Can you work these out from the model? Positions are in its coordinate system, mm. A direction names the side the tool comes from. Round coordinates to 2 decimals unless told otherwise and drop trailing zeros. Order: outer loops, then holes, each group sorted by start corner. A loop starts at its lowest first (then second) coordinate and runs counter-clockwise, first axis right, second up.
Q1. If we section it at B-B (z = 8.5): Please give me the cut outline in (x, y).
Q2. If we section it at C-C (z = -7): Please give me the cut outline in (x, y), plus the area to 3 significant figures.
Q3. If we section it at D-D (x = -14): Please give me the cut outline in (y, z), plus the area to 4 significant figures.
Q4. If I drill on line 1 (X direction, y = 2, z = 1.25); line 2 (X direction, y = 13.5, z = 13.75); line 3 (X direction, y = 18.5, z = -7.5), over which ranges is the centre line in solid material (lowest first)?
Q5. For faces 5 (the face through (-34, 14, -10.57)), 6 (the face through (32, 14, -10.57)), 7 (the face through (-25, 8, 13.82)), 8 (the face through (-2, 8, 15.57)), 9 (the face through (-18, 10, 11)), which set-ups out of +Z, -Z, +X, -X, +Y, -Y let a thin tool reach every point of the face, with its end or its side?
Q6. We'd pull the mould along X, two halves only. Please class faces 1 (the face through (30.72, 6.88, -12.05)), 2 (the face through (-2, -3, 1)), 3 (the face through (25, 10, -3.18)), 4 (the face through (-25, 8, -1.68)): pulls with the +X half, pulls with the -X half, needs draft (parallel to the pull), parting line crosses it, or undercut.
Q7. If we section it at A-A (x = 25.5): Please give me the cut outline in (y, z), plus the area to 3 significant figures.
Q8. Will these pins go through, and if not, where does the flat tip stop? P1, Ø1.3, axis at x = -23.5, y = 13.5, coming from the -Z side; P2, Ø3, axis at x = -4, z = 4.5, coming from the +Y side; P3, Ø1.3, axis at x = 20.5, y = 12.5, coming from the -Z side; P4, Ø3.5, axis at x = -35.5, y = 7, coming from the +Z side.
Autodesk Inventor part; units mm, degrees
ref_plane "YZ Plane" through (0, 0, 0) normal (1, 0, 0) x (0, 1, 0)
ref_plane "XZ Plane" through (0, 0, 0) normal (0, 1, 0) x (-1, 0, 0)
ref_plane "XY Plane" through (0, 0, 0) normal (0, 0, 1) x (1, 0, 0)
sketch "Boceto1" plane through (0, 0, 0) normal (0, 1, 0) x (-1, 0, 0)
  line L0 (24, 13.57) -> (26.5, 13.57)
  line L1 (-26.5, 13.57) -> (26.5, -13.57) construction
  line L2 (26.5, 13.57) -> (-26.5, -13.57) construction
  line L3 (24, 13.57) -> (24, 10.27) construction
  line L4 (24, 10.27) -> (20, 10.27) construction
  line L5 (20, 10.27) -> (20, 1.87) construction
  line L6 (20, 1.87) -> (24, 1.87) construction
  line L7 (24, 1.87) -> (24, -1.43) construction
  line L8 (24, -1.43) -> (26.5, -1.43) construction
  line L9 (26.75, -1.68) -> (23.75, -1.68)
  line L10 (23.75, -1.68) -> (23.75, 1.62)
  line L11 (23.75, 1.62) -> (19.5, 1.62)
  line L12 (19.5, 10.52) -> (23.75, 10.52)
  line L13 (23.75, 10.52) -> (23.75, 13.82)
  line L14 (27, 15.57) -> (0, 15.57)
  line L15 (18, 0.12) -> (22.25, 0.12)
  line L16 (22.25, 0.12) -> (22.25, -3.18)
  line L17 (22.25, -3.18) -> (26.75, -3.18)
  line L18 (18, 12.27) -> (0, 12.27)
  line L19 (19.5, 10.52) -> (18, 10.52)
  line L20 (19.5, 1.62) -> (18, 1.62)
  line L21 (27, 15.57) -> (29.75, 15.57)
  line L22 (29.75, 15.57) -> (29.75, -10.57)
  line L23 (29.75, -10.57) -> (36.3, -10.57)
  line L24 (36.3, -10.57) -> (36.3, -13.57)
  line L25 (36.3, -13.57) -> (26.75, -13.57)
  line L26 (0, 12.27) -> (0, 15.57)
  line L27 (23.75, 13.82) -> (26.75, 13.82)
  line L28 (18, 12.27) -> (18, 10.52)
  line L29 (18, 1.62) -> (18, 0.12)
  line L30 (26.75, -13.57) -> (26.75, -3.18)
  line L31 (26.75, -1.68) -> (26.75, 13.82)
  line L32 (26.5, 13.57) -> (26.5, -1.68) construction
  point P0 (0, 0)
  point P1 (23.75, 13.57)
  point P2 (0, 13.57)
  point P3 (27, -12.07)
  dimension "d1" = 27.14
  dimension "d2" = 15
  dimension "d4" = 3.3
  dimension "d5" = 4
  dimension "d6" = 3.3
  dimension "d10" = 0.25
  dimension "d11" = 0.25
  dimension "d12" = 1.5
  dimension "d16" = 3
  dimension "d17" = 29.14
  dimension "d23" = 18
  dimension "d24" = 2
  dimension "d25" = 0.25
  dimension "d27" = 15.57
  dimension "d28" = 29.75
  dimension "d29" = 3.3
  dimension "d30" = 0.25
  dimension "d31" = 20
  dimension "d32" = 6.5
  dimension "d33" = 0.25
  dimension "d34" = 4.25
  dimension "d36" = 0.25
  dimension "d51" = 36.3
extrude "Extrusión1" add sketch "Boceto1" along normal blind 20
mirror "Simetría1" about plane through (0, 0, 0) normal (1, 0, 0) of "Extrusión1"
sketch "Boceto2" plane through (0, 0, 0) normal (0, -1, 0) x (1, 0, 0)
  line L0 (18, 1.62) -> (18, 0.12)
  line L1 (18, 1.62) -> (-18, 1.62)
  line L2 (-18, 1.62) -> (-18, 0.12)
  line L3 (-18, 0.12) -> (-22.25, 0.12)
  line L4 (-22.25, 0.12) -> (-22.25, -3.18)
  line L5 (-22.25, -3.18) -> (-26.75, -3.18)
  line L6 (-26.75, -3.18) -> (-26.75, -13.57)
  line L7 (26.75, -3.18) -> (26.75, -13.57)
  line L8 (22.25, -3.18) -> (26.75, -3.18)
  line L9 (22.25, 0.12) -> (22.25, -3.18)
  line L10 (18, 0.12) -> (22.25, 0.12)
  line L11 (26.75, -13.57) -> (36.3, -13.57)
  line L12 (36.3, -13.57) -> (36.3, -10.57)
  line L13 (-36.3, -10.57) -> (-29.75, -10.57)
  line L14 (-36.3, -13.57) -> (-36.3, -10.57)
  line L15 (-26.75, -13.57) -> (-36.3, -13.57)
  line L16 (23.75, 1.62) -> (18, 1.62)
  line L17 (23.75, -1.68) -> (23.75, 1.62)
  line L18 (26.75, -1.68) -> (23.75, -1.68)
  line L19 (36.3, -10.57) -> (29.75, -10.57)
  line L20 (26.75, -1.68) -> (29.75, -1.68)
  line L21 (29.75, -10.57) -> (29.75, 15.57)
  line L22 (-23.75, 1.62) -> (-18, 1.62)
  line L23 (-23.75, -1.68) -> (-23.75, 1.62)
  line L24 (-26.75, -1.68) -> (-23.75, -1.68)
  line L25 (-26.75, 13.82) -> (-26.75, -1.68)
  line L26 (-26.75, -1.68) -> (-29.75, -1.68)
  line L27 (-29.75, -10.57) -> (-29.75, 15.57)
  line L28 (26.75, -13.57) -> (-26.75, -13.57)
  line L29 (-18, 12.27) -> (18, 12.27)
  line L30 (12.75, 12.27) -> (12.75, 1.62)
  line L31 (26.75, 13.82) -> (26.75, -1.68)
  line L32 (-29.75, 15.57) -> (29.75, 15.57)
  line L33 (-16.75, 12.27) -> (-16.75, 1.62)
  line L34 (23.75, 13.82) -> (26.75, 13.82)
  line L35 (18, 10.52) -> (23.75, 10.52)
  line L36 (23.75, 10.52) -> (23.75, 13.82)
  line L37 (18, 12.27) -> (18, 10.52)
  line L38 (-23.75, 10.52) -> (-23.75, 13.82)
  line L39 (-18, 10.52) -> (-23.75, 10.52)
  line L40 (-18, 12.27) -> (-18, 10.52)
  line L41 (-18, 12.27) -> (18, 12.27)
  line L42 (18, 12.27) -> (18, 10.52)
  line L43 (18, 10.52) -> (23.75, 10.52)
  line L44 (23.75, 10.52) -> (23.75, 13.82)
  line L45 (23.75, 13.82) -> (26.75, 13.82)
  line L46 (26.75, 13.82) -> (26.75, -1.68)
  line L47 (26.75, -1.68) -> (23.75, -1.68)
  line L48 (23.75, -1.68) -> (23.75, 1.62)
  line L49 (23.75, 1.62) -> (18, 1.62)
  line L50 (18, 1.62) -> (18, 0.12)
  line L51 (18, 0.12) -> (22.25, 0.12)
  line L52 (22.25, 0.12) -> (22.25, -3.18)
  line L53 (22.25, -3.18) -> (26.75, -3.18)
  line L54 (26.75, -3.18) -> (26.75, -13.57)
  line L55 (26.75, -13.57) -> (36.3, -13.57)
  line L56 (36.3, -13.57) -> (36.3, -10.57)
  line L57 (36.3, -10.57) -> (29.75, -10.57)
  line L58 (29.75, -10.57) -> (29.75, 15.57)
  line L59 (-29.75, 15.57) -> (29.75, 15.57)
  line L60 (-29.75, -10.57) -> (-29.75, 15.57)
  line L61 (-36.3, -10.57) -> (-29.75, -10.57)
  line L62 (-36.3, -13.57) -> (-36.3, -10.57)
  line L63 (-26.75, -13.57) -> (-36.3, -13.57)
  line L64 (-26.75, -3.18) -> (-26.75, -13.57)
  line L65 (-22.25, -3.18) -> (-26.75, -3.18)
  line L66 (-22.25, 0.12) -> (-22.25, -3.18)
  line L67 (-18, 0.12) -> (-22.25, 0.12)
  line L68 (-18, 1.62) -> (-18, 0.12)
  line L69 (-23.75, 1.62) -> (-18, 1.62)
  line L70 (-23.75, -1.68) -> (-23.75, 1.62)
  line L71 (-26.75, -1.68) -> (-23.75, -1.68)
  line L72 (-26.75, 13.82) -> (-26.75, -1.68)
  line L73 (-23.75, 13.82) -> (-26.75, 13.82)
  line L74 (18, 10.52) -> (12.75, 10.52)
  line L75 (-18, 10.52) -> (-16.75, 10.52)
  point P0 (0, 0)
  point P1 (0, 1.62)
  point P2 (12.75, 12.27)
  dimension "d42" = 14
  dimension "d43" = 10
extrude "Extrusión2" add sketch "Boceto2" along normal blind 3 contours L16 L17 L18 L20 L21 L19 L12 L11 L7 L8 L9 L10 L0 | L0 L10 L9 L8 L7 L28 L6 L5 L4 L3 L2 L1 | L1 L33 L29 L30 | L30 L29 L37 L74 | L2 L3 L4 L5 L6 L15 L14 L13 L27 L26 L24 L23 L22 | L75 L40 L29 L33 | L29 L40 L39 L38 L73 L25 L26 L27 L32 L21 L20 L31 L34 L36 L35 L37
move faces "Desplazar2" translate (0, -0.5, 0) faces at (4.25, 0, -8.5067)
move faces "Desplazar3" translate (-1.1, 0, 0) faces at (-29.75, 12.3333, 6.8567)
move faces "Desplazar4" translate (-1.1, 0, 0) faces at (29.75, 12.3333, 6.8567)
move faces "Desplazar5" translate (-2, 0, 0) faces at (-36.3, 12.3333, -11.57)
sketch "Boceto5" plane through (-36.3, -3, -10.57) normal (0, 0, 1) x (1, 0, 0)
  line L0 (0, 0) -> (72.6, 0)
  line L1 (5.45, 0) -> (5.45, 23)
  line L2 (0, 0) -> (5.45, 0)
  line L3 (5.45, 0) -> (5.45, 16.75)
  line L4 (5.45, 16.75) -> (-2, 16.75)
  line L5 (-2, 16.75) -> (-2, 0)
  line L6 (64.95, 23) -> (64.95, 0)
  line L7 (64.95, 0) -> (72.6, 0)
  line L8 (72.6, 0) -> (72.6, 16.75)
  line L9 (72.6, 16.75) -> (64.95, 16.75)
  line L10 (64.95, 16.75) -> (64.95, 0)
  line L11 (72.6, 23) -> (64.95, 23)
  line L12 (5.45, 0) -> (-2, 0)
  point P0 (36.3, 3)
  dimension "d63" = 6.25
extrude "Extrusión5" cut sketch "Boceto5" against normal blind 10
fillet "Empalme2" radius 20 2 edges at (28.65, 13.75, -12.07) (-30.85, 13.75, -12.07)
sketch "Boceto7" plane through (36.3, 20, -13.57) normal (0, 0, -1) x (-1, 0, 0)
  line L0 (65.05, -19) -> (63.05, -19)
  line L1 (63.05, -19) -> (63.05, -1)
  line L2 (63.05, -1) -> (65.05, -1)
  line L3 (65.05, -1) -> (65.05, -19)
  line L4 (63.05, -20.5) -> (9.55, -20.5)
  line L5 (63.05, -20.5) -> (63.05, 0)
  point P0 (36.3, -20)
  dimension "d75" = 2
  dimension "d76" = 18
  dimension "d77" = 1.5
extrude "Extrusión7" cut sketch "Boceto7" against normal blind 3
sketch "Boceto8" plane through (-38.3, 20, -10.57) normal (0, 0, 1) x (1, 0, 0)
  circle A0 centre (4.175, -3.125) radius 2
  circle A1 centre (70.225, -3.125) radius 2
  circle A2 centre (4.175, -3.125) radius 3
  circle A3 centre (70.225, -3.125) radius 3
  point P0 (38.3, -20)
  dimension "d80" = 6
  dimension "d81" = 6
extrude "Extrusión8" cut sketch "Boceto8" against normal through all contours A0 | A1
equation "\"d6\" = d4"
equation "\"d9\" = d7"
properties part number "Guía" material "Plástico PC/ABS"
Solution:
1. outline: (-30.85, -3) - (-26.75, -3) - (-26.75, 20) - (-30.85, 20) - close; (-16.75, -3) - (12.75, -3) - (12.75, -0.5) - (-16.75, -0.5) - close; (26.75, -3) - (28.65, -3) - (28.65, 20) - (26.75, 20) - close
2. outline: (-30.85, -3) - (28.65, -3) - (28.65, 20) - (26.75, 20) - (26.75, -0.5) - (-26.75, -0.5) - (-26.75, 20) - (-30.85, 20) - close
2. area: 272 mm2
3. outline: (-3, -13.57) - (-0.5, -13.57) - (-0.5, 12.27) - (20, 12.27) - (20, 15.57) - (-3, 15.57) - close
3. area: 140.5 mm2
4. line 1: x = -30.85 to -26.75, -23.75 to -18, 18 to 23.75, 26.75 to 28.65
4. line 2: x = -30.85 to -26.75, -23.75 to 23.75, 26.75 to 28.65
4. line 3: x = -30.85 to -26.75, 26.75 to 28.65
5. face 5: +Z, -X, +Y, -Y
5. face 6: +Z, +X, +Y, -Y
5. face 7: +Y, -Y
5. face 8: +Z, +X, -X, +Y, -Y
5. face 9: -Z, +Y
6. face 1: pulls with the +X half
6. face 2: needs draft
6. face 3: undercut
6. face 4: undercut
7. outline: (-3, -13.57) - (-0.5, -13.57) - (-0.5, -3.18) - (20, -3.18) - (20, -1.68) - (-3, -1.68) - close; (-3, 13.82) - (20, 13.82) - (20, 15.57) - (-3, 15.57) - close
7. area: 101 mm2
8. P1: stops at z = -3.18
8. P2: stops at y = -0.5
8. P3: stops at z = 0.12
8. P4: passes through
